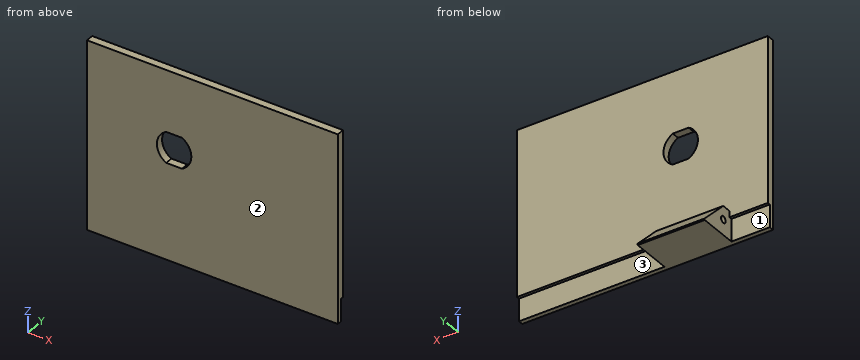
from build123d import *

# Parameters (mm, degrees)
SKETCH1_W               = 131
SKETCH1_H               = 98
BOSS_EXTRUDE1_DEPTH     = 4
LOCK_HOLE_DEPTH         = 82.897802168
SKETCH6_W               = 11.75
SKETCH6_H               = 1.5
CUT_EXTRUDE4_DEPTH      = 131
SKETCH3_W               = 35
SKETCH3_H               = 15
BOSS_EXTRUDE2_DEPTH     = 19
SKETCH4_R               = 1.75
CUT_EXTRUDE2_DEPTH      = 35
CUT_EXTRUDE3_DEPTH      = 124.494939168
CUT_EXTRUDE3_DEPTH_BACK = 124.494939168
SKETCH7_W               = 35
SKETCH7_H               = 1.5
BOSS_EXTRUDE3_DEPTH     = 11.75


with BuildPart() as part:
    # Sketch1 → Boss-Extrude1 (new body)
    with BuildSketch(Plane(origin=(0, 0, 0), x_dir=(1, 0, 0), z_dir=(0, 1, 0))):
        Rectangle(SKETCH1_W, SKETCH1_H)
    extrude(amount=BOSS_EXTRUDE1_DEPTH)

    # Lock → Lock Hole (cut, through all)
    with BuildSketch(Plane(origin=(0, 4, 0), x_dir=(1, 0, 0), z_dir=(0, 1, 0))):
        with BuildLine():
            Line((-24.123105626, -1), (-15.876894374, -1))
            ThreePointArc((-15.876894374, -1), (-11, -9), (-15.876894374, -17))
            Line((-15.876894374, -17), (-24.123105626, -17))
            ThreePointArc((-24.123105626, -17), (-29, -9), (-24.123105626, -1))
        make_face()
    extrude(amount=-LOCK_HOLE_DEPTH, mode=Mode.SUBTRACT)

    # Sketch6 → Cut-Extrude4 (cut)
    with BuildSketch(Plane.ZY.offset(65.5)):
        with Locations((-43.125, 3.25)):
            Rectangle(SKETCH6_W, SKETCH6_H)
    extrude(amount=-CUT_EXTRUDE4_DEPTH, mode=Mode.SUBTRACT)

    # Sketch3 → Boss-Extrude2 (add)
    with BuildSketch(Plane(origin=(0, 4, 0), x_dir=(1, 0, 0), z_dir=(0, 1, 0))):
        with Locations((-28, 41.5)):
            Rectangle(SKETCH3_W, SKETCH3_H)
    extrude(amount=BOSS_EXTRUDE2_DEPTH)

    # Sketch4 → Cut-Extrude2 (cut)
    with BuildSketch(Plane.ZY.offset(45.5)):
        with Locations((-41, 8.75)):
            Circle(SKETCH4_R)
    extrude(amount=-CUT_EXTRUDE2_DEPTH, mode=Mode.SUBTRACT)

    # Sketch5 → Cut-Extrude3 (cut, two sides: drawn at the far end of the back side and taken through both)
    with BuildSketch(Plane.ZY.offset(45.5).offset(-CUT_EXTRUDE3_DEPTH_BACK)):
        Polygon((-34, 8.811703297), (-48.188296703, 23), (-34, 23), align=None)
    extrude(amount=CUT_EXTRUDE3_DEPTH + CUT_EXTRUDE3_DEPTH_BACK, mode=Mode.SUBTRACT)

    # Sketch7 → Boss-Extrude3 (add)
    with BuildSketch(Plane(origin=(0, 0, -49), x_dir=(-1, 0, 0), z_dir=(0, 0, -1))):
        with Locations((28, 3.25)):
            Rectangle(SKETCH7_W, SKETCH7_H)
    extrude(amount=-BOSS_EXTRUDE3_DEPTH)


solid = part.part
Design review of the part built by this model. Coordinates are the model's own, in mm. Face numbers are marked on the shaded views. A direction names the side the tool comes from. Coordinates: 2 decimals unless noted, no trailing zeros. Order: outer loops, then holes, each group sorted by start corner. A loop starts at its lowest first (then second) coordinate and runs counter-clockwise, first axis right, second up. Notation, with made-up numbers: (-35.5, 45.5) -> (-24.5, 45.5) arc R19 cw to (-24.5, 81.5) -> close; hole circle Ø4 at (-33, 59). An arc over 180 degrees is marked (long way). One line per item, written item: value.
1) We need section D-D, the plane z = 28. Give the boundary of the cut face in (x, y), then the cut area to 3 significant figures.
Output values:
outline: (-65.5, 0) -> (65.5, 0) -> (65.5, 4) -> (-65.5, 4) -> close
area: 524 mm2
2) To check wall thickness, follow probe 1 along Y at (x, z) = (-33.5, -41); probe 2 along Y at (x, z) = (-14, 29); probe 3 along Z at (x, y) = (-36.5, 15). State the ranges of each line that lie inside material, in increasing order. Write a range as [from, to].
Output values:
probe 1: y = [0, 7], [10.5, 15.81]
probe 2: y = [0, 4]
probe 3: z = [-49, -40.19]
3) We need section B-B, the plane z = -41. Give the boundary of the cut face in (x, y), then the cut area to 3 significant figures.
Output values:
outline: (-65.5, 0) -> (65.5, 0) -> (65.5, 2.5) -> (-10.5, 2.5) -> (-10.5, 7) -> (-45.5, 7) -> (-45.5, 2.5) -> (-65.5, 2.5) -> close; (-45.5, 10.5) -> (-10.5, 10.5) -> (-10.5, 15.81) -> (-45.5, 15.81) -> close
area: 671 mm2
4) We need section A-A, the plane x = -42. Give the boundary of the cut face in (y, z), then the cut area to 3 significant figures.
Output values:
outline: (0, -49) -> (23, -49) -> (23, -48.19) -> (8.81, -34) -> (4, -34) -> (4, 49) -> (0, 49) -> close; hole circle Ø3.5 at (8.75, -41)
area: 567 mm2
5) Clearance check with flat-ended pins moving along their axes: P1, Ø12, axis at y = 17.5, z = -43, coming from the -X side; P2, Ø4, axis at x = 37, z = -28.5, coming from the +Y side; P3, Ø13, axis at x = -60.5, z = -44.5, coming from the +Y side. State where each tip first meets the part, or that it passes through.
Output values:
P1: stops at x = -45.5
P2: stops at y = 4
P3: stops at y = 2.5
6) Machinability: for the marked faces 1, 2 and 3, which of the approach directions +Z, -Z, +X, -X, +Y, -Y give a long, thin tool a straight path to every point of the face, cutting with its end or side? Answer none if there is none.
Output values:
face 1: -Z, -X, +Y
face 2: +Z, -Z, +X, -X, -Y
face 3: -Z, +X, +Y
7) We need section C-C, the plane y = 13.25. Give the boundary of the cut face in (x, z).
Output values:
outline: (-45.5, -49) -> (-10.5, -49) -> (-10.5, -38.44) -> (-45.5, -38.44) -> close
